Geometry check sheet. Reference: the model listing, model coordinates, mm. Face numbers are marked on the shaded views. A direction names the side the tool comes from. Give positions to 0.01 mm unless a question says otherwise; leave off trailing zeros. Order: outer loops, then holes, each group sorted by start corner. A loop starts at its lowest first (then second) coordinate and runs counter-clockwise, first axis right, second up. Notation, with made-up numbers: M 56.25,-7 L 91.25,-7 A18 cw 91.25,18 Z; hole C -32.75,-15.5 d6. An arc over 180 degrees is marked long. Put each result on its own line as item: value. Start each with the question number.
Q1. Go/stop test with flat-tipped pins: pin 1 (0.5 mm diameter, centred on x = -1.5, z = 4.5, fed in from -Y); pin 2 (4 mm diameter, centred on y = -7, z = 2.5, fed in from -X); pin 3 (0.9 mm diameter, centred on x = 2, z = 3.5, fed in from -Y); pin 4 (4 mm diameter, centred on y = -9, z = 1.5, fed in from +X). Record where each tip stops, or that it passes through.
Q2. Access from +Z, -Z, +X, -X, +Y, -Y to the whole of each face (thin tool, end or side, straight path). Record for the marked faces 1, 2, 3 and 4.
Q3. Section check C-C on z = 4. Record the cut outline in (x, y) (3 decimals), then the cut area to 3 significant figures.
Q4. Material ranges on L1, parallel to X at y = 0, z = 7.25 (3 decimals); L2, parallel to Y at x = 0, z = 10.5 (3 decimals); L3, parallel to X at y = -3, z = 4 (3 decimals), recorded low to high.
Q5. Section check D-D on y = -3.75. Record the cut outline in (x, z) (3 decimals).
Q6. Section check B-B on y = -5.75. Record the cut outline in (x, z).
Q7. Mould release check, pull along Y, two halves, no side actions. Record for the marked faces 5, 6 and 7: +Y half, -Y half, draft (parallel to the pull), parting line (faces both ways), or undercut.
Q8. Section check A-A on x = 0. Record the cut outline in (y, z) (3 decimals).
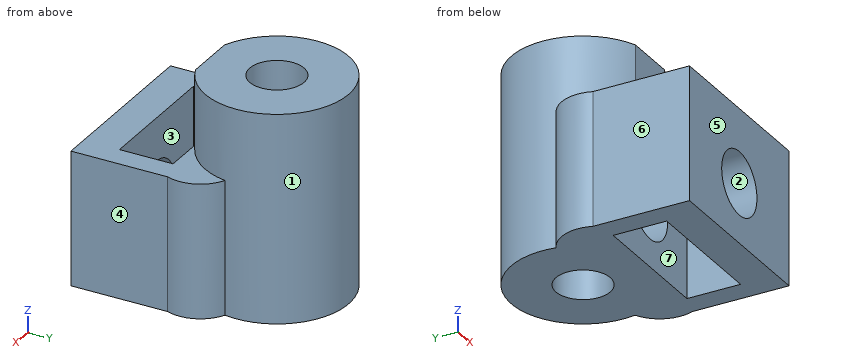
Autodesk Inventor part; units mm, degrees
ref_plane "Work Plane1" through (0, -10.5, 0) normal (0, 1, 0) x (-1, 0, 0)
ref_plane "YZ Plane" through (0, 0, 0) normal (1, 0, 0) x (0, 1, 0)
ref_plane "XY Plane" through (0, 0, 0) normal (0, 0, 1) x (1, 0, 0)
sketch "Sketch1" plane through (0, 0, 0) normal (0, 0, 1) x (1, 0, 0)
  circle A0 centre (0, 0) radius 1.825
  circle A1 centre (0, 0) radius 4.825
  line L0 (-6, -4) -> (6, -4)
  line L1 (6, -10.5) -> (-6, -10.5)
  line L2 (-6, -10.5) -> (-6, -4)
  arc A2 (-2.3662, -0.949) -> (-6, -4) centre (-3.6609, -3.0965) ccw
  arc A3 (6, -4) -> (2.3662, -0.949) centre (3.6609, -3.0965) ccw
  arc A4 (-2.3662, -0.949) -> (2.3662, -0.949) centre (0, 0.4878) ccw
  line L3 (-15.4666, 0) -> (16.043, 0) construction
  line L4 (0, 8.2762) -> (0, -10.4238) construction
  line L5 (6, -10.5) -> (6, -4)
  dimension "d0" = 3.65
  dimension "d1" = 3
  dimension "d3" = 12
  dimension "d5" = 4
  dimension "d6" = 6.5
  dimension "d7" = 6
extrude "Extrusion1" add sketch "Sketch1" along normal blind 9
ref_plane "Work Plane1" through (0, -10.5, 0) normal (0, 1, 0) x (-1, 0, 0)
extrude "Extrusion4" add sketch "Sketch1" along normal blind 14 contours A1 A3 A4 A2 | A2 A4 A3 A1 L0 | L0 A1
sketch "Sketch2" plane through (0, -10.5, 0) normal (0, 1, 0) x (-1, 0, 0)
  line L0 (6, 0) -> (-6, 0)
  line L1 (-6, 0) -> (-6, 9)
  line L2 (6, 9) -> (-6, 9)
  line L3 (6, 0) -> (6, 9)
  circle A0 centre (0, 4) radius 2.125
  point P0 (0, 0)
  dimension "d11" = 4.25
  dimension "d12" = 4
extrude "Extrusion2" cut sketch "Sketch2" along normal blind 12 contours A0
sketch "Sketch3" plane through (0, 0, 9) normal (0, 0, 1) x (1, 0, 0)
  line L0 (-6, -10.5) -> (6, -10.5)
  circle A0 centre (0, 0) radius 1.825
  line L1 (-4.45, -4.5) -> (4.45, -4.5)
  line L2 (4.45, -4.5) -> (4.45, -8.1)
  line L3 (4.45, -8.1) -> (-4.45, -8.1)
  line L4 (-4.45, -8.1) -> (-4.45, -4.5)
  point P0 (0, -8.1)
  point P1 (0, -10.5)
  dimension "d15" = 8.9
  dimension "d16" = 3.6
  dimension "d17" = 4.5
extrude "Extrusion3" cut sketch "Sketch3" along normal mid plane 30 contours L1 L2 L3 L4
equation "\"d4\" = 0.4"
properties part number "MotorAttachment2"
Results found:
1. pin 1: stops at y = 1.5
1. pin 2: stops at x = -6
1. pin 3: stops at y = -10.5
1. pin 4: stops at x = 6
2. face 1: +Z
2. face 2: -Y
2. face 3: +Z, -Z
2. face 4: +Z, -Z, +X, -Y
3. outline: M -6,-10.5 L -2.125,-10.5 L -2.125,-8.1 L -4.45,-8.1 L -4.45,-4.5 L -2.125,-4.5 L -2.125,1.5 L -1.04,1.5 A1.825 cw 1.04,1.5 L 2.125,1.5 L 2.125,-4.5 L 4.45,-4.5 L 4.45,-8.1 L 2.125,-8.1 L 2.125,-10.5 L 6,-10.5 L 6,-4 A2.508 ccw 4.752,-0.839 A4.825 ccw long -4.752,-0.839 A2.508 ccw -6,-4 Z
3. area: 91.5 mm^2
4. L1: x = -4.825 to -1.825, 1.825 to 4.825
4. L2: y = -4.5 to -1.825, 1.825 to 4.825
4. L3: x = -6.167 to -2.125, 2.125 to 6.167
5. outline: M -6.082,0 L 6.082,0 L 6.082,9 L 3.036,9 L 3.036,14 L -3.036,14 L -3.036,9 L -6.082,9 Z; hole C 0,4 d4.25
6. outline: M -6,0 L -4.45,0 L -4.45,9 L -6,9 Z; M 4.45,0 L 6,0 L 6,9 L 4.45,9 Z
7. face 5: -Y half
7. face 6: draft
7. face 7: undercut
8. outline: M -10.5,0 L -8.1,0 L -8.1,1.875 L -10.5,1.875 Z; M -10.5,6.125 L -8.1,6.125 L -8.1,9 L -10.5,9 Z; M -4.5,0 L -1.825,0 L -1.825,1.875 L -4.5,1.875 Z; M -4.5,6.125 L -1.825,6.125 L -1.825,14 L -4.5,14 Z; M 1.825,0 L 4.825,0 L 4.825,14 L 1.825,14 Z
